Geometry check sheet. Reference: drawing and pictorial views, mm from the part's lowest x, y, z. Give positions to 0.01 mm unless a question says otherwise; leave off trailing zeros. Loops run counter-clockwise (first coordinate to the right, second up) from the corner with the lowest first, then second, coordinate; pieces in that order, holes last. Notation, with made-up numbers: (84.25, -1) -> (142.25, -1) arc R21 cw to (142.25, 35) -> close; hole circle Ø1 at (82.5, 44.5). An arc over 180 degrees is marked (long way). Answer in a Markdown table with one row per item. Add a question column.
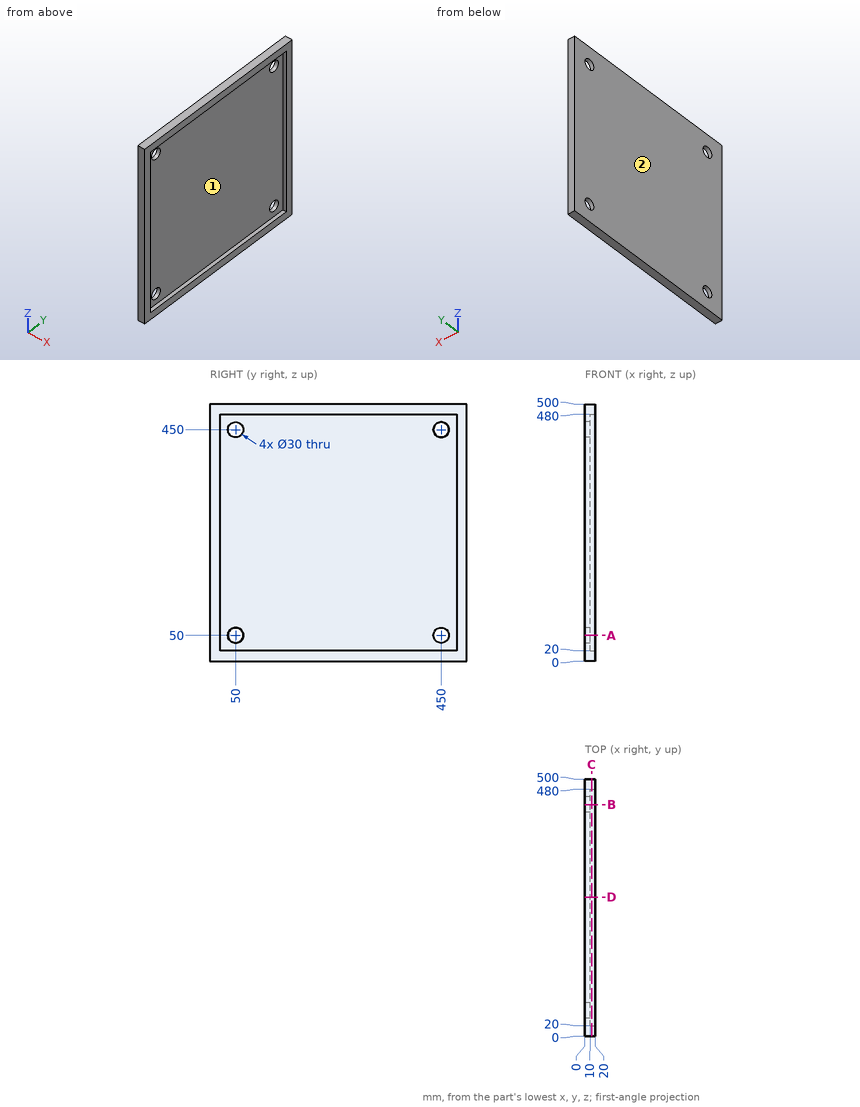
1. Release check for a two-part mould opening along Y. For the marked faces 1 and 2 record: released by +Y, released by -Y, zero draft, split by the parting line, or undercut.
2. Gauge pin test, flat end, axial feed: pin 1 Ø1.5 at (y, z) = (378, 215) entering from +X. Record the tip position at first contact, or that the pin passes through.
3. Sectioned sample at A-A (z = 50). Enter the section's corners in (x, y), plus the area to 3 significant figures.
4. Sectioned sample at C-C (x = 13). Enter the section's corners in (y, z).
5. Material ranges on L1, parallel to Y at x = 6, z = 450; L2, parallel to Y at x = 18.5, z = 372, recorded low to high. Write a range as from..to.
6. Sectioned sample at D-D (y = 270). Enter the section's corners in (x, z).
Response:
| question | item | result |
|---|---|---|
| 1 | face 1 | undercut |
| 1 | face 2 | zero draft |
| 2 | pin 1 | stops at x = 10 |
| 3 | outline | (0, 0) -> (20, 0) -> (20, 20) -> (10, 20) -> (10, 35) -> (0, 35) -> close; (0, 65) -> (10, 65) -> (10, 435) -> (0, 435) -> close; (0, 465) -> (10, 465) -> (10, 480) -> (20, 480) -> (20, 500) -> (0, 500) -> close |
| 3 | area | 4,800 mm2 |
| 4 | outline | (0, 0) -> (500, 0) -> (500, 500) -> (0, 500) -> close; hole (20, 20) -> (480, 20) -> (480, 480) -> (20, 480) -> close |
| 5 | L1 | y = 0..35, 65..435, 465..500 |
| 5 | L2 | y = 0..20, 480..500 |
| 6 | outline | (0, 0) -> (20, 0) -> (20, 20) -> (10, 20) -> (10, 480) -> (20, 480) -> (20, 500) -> (0, 500) -> close |
